from build123d import *

# Parameters (mm, degrees)
F0_R            = 62.5
F1_DEPTH        = 12
F2_R            = 7
F3_DEPTH        = 7
F3_COPIES_COUNT = 4
F4_R            = 4
F5_DEPTH        = 25
F5_COPIES_COUNT = 4
F7_DEPTH        = 25
F8_R            = 42.5
F9_DEPTH        = 13
F10_R           = 35
F11_DEPTH       = 8
F12_R           = 34
F13_DEPTH       = 11
F14_R           = 30
F15_DEPTH       = 25
F16_SIZE        = 1
F17_R           = 0.5
F18_R           = 3


# Not quite as in the source:
# - a pattern or mirror of a feature is missing from the dataset's text; its kind, count and spacing are read off the source's solid


with BuildPart() as f1:
    # F0 (on Front) → F1 (new body)
    with BuildSketch(Plane.XZ):
        Circle(F0_R)
    extrude(amount=-F1_DEPTH)

    # F2 (on face) → F3 (cut)
    with BuildSketch(Plane.XZ):
        with Locations((37.1231060123, 37.1231060123)):
            Circle(F2_R)
    f3 = extrude(amount=-F3_DEPTH, mode=Mode.SUBTRACT)

    # F3_copies: F3 ×4 about axis
    f3_copies_axis = Axis((0, 0, 0), (0, 1, 0))
    for i in range(1, F3_COPIES_COUNT):
        add(f3.rotate(f3_copies_axis, i * 360 / F3_COPIES_COUNT), mode=Mode.SUBTRACT)

    # F4 (on face) → F5 (cut)
    with BuildSketch(Plane.XZ.offset(-7)):
        with Locations((37.1231060123, 37.1231060123)):
            Circle(F4_R)
    f5 = extrude(amount=-F5_DEPTH, mode=Mode.SUBTRACT)

    # F5_copies: F5 ×4 about axis
    f5_copies_axis = Axis((0, 0, 0), (0, 1, 0))
    for i in range(1, F5_COPIES_COUNT):
        add(f5.rotate(f5_copies_axis, i * 360 / F5_COPIES_COUNT), mode=Mode.SUBTRACT)

    # F6 (on face) → F7 (cut)
    with BuildSketch(Plane.XZ):
        with BuildLine():
            Line((30.5941170816, -54.5), (-30.5941170816, -54.5))
            ThreePointArc((-30.5941170816, -54.5), (0, -62.5), (30.5941170816, -54.5))
        make_face()
    extrude(amount=-F7_DEPTH, mode=Mode.SUBTRACT)

    # F8 (on face) → F9 (join)
    with BuildSketch(Plane(origin=(0, 12, 0), x_dir=(-1, 0, 0), z_dir=(0, 1, 0))):
        Circle(F8_R)
    extrude(amount=F9_DEPTH)

    # F10 (on face) → F11 (cut)
    with BuildSketch(Plane(origin=(0, 25, 0), x_dir=(-1, 0, 0), z_dir=(0, 1, 0))):
        Circle(F10_R)
    extrude(amount=-F11_DEPTH, mode=Mode.SUBTRACT)

    # F12 (on face) → F13 (cut)
    with BuildSketch(Plane.XZ):
        Circle(F12_R)
    extrude(amount=-F13_DEPTH, mode=Mode.SUBTRACT)

    # F14 (on face) → F15 (cut)
    with BuildSketch(Plane.XZ.offset(-11)):
        Circle(F14_R)
    extrude(amount=-F15_DEPTH, mode=Mode.SUBTRACT)

    # F16
    f16_edges = [f1.edges().sort_by_distance(p)[0] for p in [
        (0, 0, 62.5),
        (-34, 0, 0),
        (42.5, 25, 0),
    ]]
    chamfer(f16_edges, length=F16_SIZE)

    # F17
    f17_edges = [f1.edges().sort_by_distance(p)[0] for p in [
        (-34, 11, 0),
        (42.5, 12, 0),
    ]]
    fillet(f17_edges, radius=F17_R)

    # F18
    f18_edges = [f1.edges().sort_by_distance(p)[0] for p in [
        (35, 17, 0),
    ]]
    fillet(f18_edges, radius=F18_R)


with BuildPart() as f20:
    # F19 (on Top) → F20 (revolve)
    with BuildSketch(Plane.XY):
        with BuildLine():
            Line((23, 17), (23, 0))
            Line((23, 0), (34, 0))
            Line((34, 0), (34, 10.5))
            ThreePointArc((34, 10.5), (33.8535533906, 10.8535533906), (33.5, 11))
            Line((33.5, 11), (30, 11))
            Line((30, 11), (30, 17))
            Line((30, 17), (23, 17))
        make_face()
    revolve(axis=Axis((0, 0, 0), (0, -1, 0)))


solid = f1.part
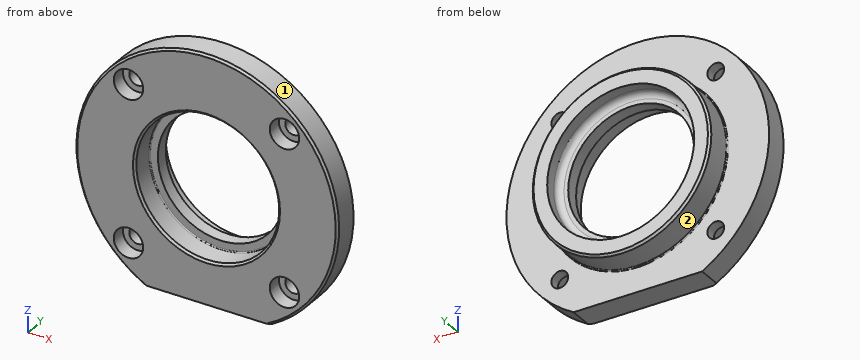
Geometry check sheet. Reference: the model listing, model coordinates, mm. Face numbers are marked on the shaded views. A direction names the side the tool comes from. Give positions to 0.01 mm unless a question says otherwise; leave off trailing zeros. Use a Markdown table: item, result.
Item 1: Depth check by flat-ended pin: P1, Ø12.5, axis at x = 37.12, z = 37.12, coming from the +Y side; P2, Ø6, axis at x = 12.5, z = -26, coming from the -Y side; P3, Ø3, axis at y = 20.5, z = 6.5, coming from the -X side. Enter the tip coordinate at first touch or a pass-through.
Answers follow:
| item | result |
|---|---|
| P1 | stops at y = 12 |
| P2 | stops at y = 11 |
| P3 | stops at x = -42.2 |
Item 2: Material ranges on line 1 along Y through (x, z) = (44.5, -32.5); line 2 along X through (y, z) = (5.25, -8); line 3 along X through (y, z) = (23, 4.5), recorded low to high.
Answers follow:
| item | result |
|---|---|
| line 1 | y = 0 to 12 |
| line 2 | x = -61.99 to -33.05, 33.05 to 61.99 |
| line 3 | x = -42.26 to -34.71, 34.71 to 42.26 |
Item 3: Tool access check on the marked faces 1 and 2. Record the directions out of +Z, -Z, +X, -X, +Y, -Y that give a thin tool (end or side, any length) a straight path to the whole face; none if there is none.
Answers follow:
| item | result |
|---|---|
| face 1 | +Y, -Y |
| face 2 | +Y |
